For this review, take the finished solid that the model builds, in its own axes (mm). Face numbers are marked on the shaded views. A direction names the side the tool comes from. Give positions to 0.01 mm unless a question says otherwise; leave off trailing zeros. Loops run counter-clockwise (first coordinate to the right, second up) from the corner with the lowest first, then second, coordinate; pieces in that order, holes last. Notation, with made-up numbers: (-17.75, -30) - (-11.75, -30) arc R20 cw to (-11.75, -5) - close; hole circle Ø9 at (40.5, 88). An arc over 180 degrees is marked (long way). Answer in a Markdown table with one row per item.
```python
from build123d import *

# Parameters (mm, degrees)
F0_W      = 10
F0_H      = 3.5
F1_DEPTH  = 20
F2_R      = 3
F3_DEPTH  = 3.501
F6_R      = 5
F9_DEPTH  = 19
F10_DEPTH = 5
F11_R     = 5


with BuildPart() as f1:
    # F0 (on Front) → F1 (new body)
    with BuildSketch(Plane.XZ):
        with Locations((-70, 1.75)):
            Rectangle(F0_W, F0_H)
        Polygon((-65, 0), (0, 0), (0, 3.5), (0, 32), (-65, 32), (-65, 3.5), align=None)
        with Locations((5, 1.75)):
            Rectangle(F0_W, F0_H)
    extrude(amount=F1_DEPTH)

    # F2 (on face) → F3 (cut, through all)
    with BuildSketch(Plane.XY.offset(3.5)):
        with Locations((5, -10)):
            Circle(F2_R)
    f3 = extrude(amount=-F3_DEPTH, mode=Mode.SUBTRACT)

    # F5: F3 across plane
    add(f3.mirror(Plane.YZ.offset(-32.5)), mode=Mode.SUBTRACT)

    # F6
    f6_edges = [f1.edges().sort_by_distance(p)[0] for p in [
        (0, -10, 32),
        (-65, -10, 32),
    ]]
    fillet(f6_edges, radius=F6_R)

    # F8 (on face) → F9 (cut)
    with BuildSketch(Plane.XZ.offset(20)):
        with BuildLine():
            Line((-58.5, 2.5), (-6.5, 2.5))
            ThreePointArc((-6.5, 2.5), (-5.0857864376, 3.0857864376), (-4.5, 4.5))
            Line((-4.5, 4.5), (-4.5, 27.5))
            ThreePointArc((-4.5, 27.5), (-5.0857864376, 28.9142135624), (-6.5, 29.5))
            Line((-6.5, 29.5), (-58.5, 29.5))
            ThreePointArc((-58.5, 29.5), (-59.9142135624, 28.9142135624), (-60.5, 27.5))
            Line((-60.5, 27.5), (-60.5, 4.5))
            ThreePointArc((-60.5, 4.5), (-59.9142135624, 3.0857864376), (-58.5, 2.5))
        make_face()
    extrude(amount=-F9_DEPTH, mode=Mode.SUBTRACT)

    # F7 (on face) → F10 (cut)
    with BuildSketch(Plane(origin=(0, 0, 0), x_dir=(-1, 0, 0), z_dir=(0, 1, 0))):
        with BuildLine():
            Line((7.5, 4), (57.5, 4))
            ThreePointArc((57.5, 4), (58.9142135624, 4.5857864376), (59.5, 6))
            Line((59.5, 6), (59.5, 26))
            ThreePointArc((59.5, 26), (58.9142135624, 27.4142135624), (57.5, 28))
            Line((57.5, 28), (7.5, 28))
            ThreePointArc((7.5, 28), (6.0857864376, 27.4142135624), (5.5, 26))
            Line((5.5, 26), (5.5, 6))
            ThreePointArc((5.5, 6), (6.0857864376, 4.5857864376), (7.5, 4))
        make_face()
    extrude(amount=-F10_DEPTH, mode=Mode.SUBTRACT)

    # F11
    f11_edges = [f1.edges().sort_by_distance(p)[0] for p in [
        (-75, -20, 1.75),
        (-75, 0, 1.75),
        (10, -20, 1.75),
        (10, 0, 1.75),
    ]]
    fillet(f11_edges, radius=F11_R)


solid = f1.part
```
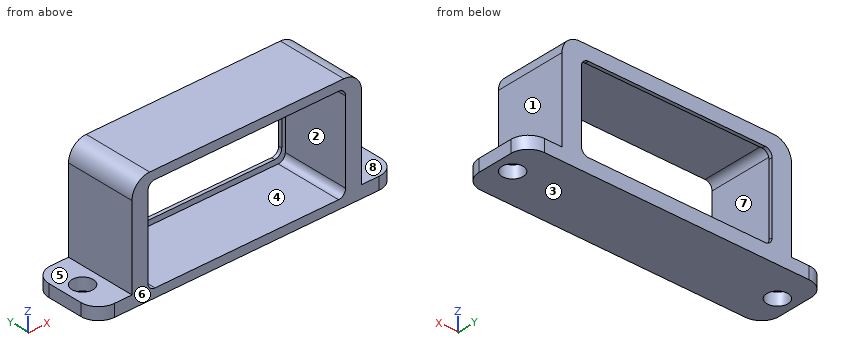
1. Mouldability with a two-part tool opening along Z and no side actions: class the marked faces 1, 2, 3 and 4 as released by +Z, released by -Z, zero draft, split by the parting line, or undercut.
Values:
| item | result |
|---|---|
| face 1 | zero draft |
| face 2 | undercut |
| face 3 | released by -Z |
| face 4 | undercut |
2. We need section A-A, the plane y = -9.25. Give the boundary of the cut face in (x, z).
Values:
| item | result |
|---|---|
| outline | (-75, 0) - (-72.9, 0) - (-72.9, 3.5) - (-75, 3.5) - close; (-67.1, 0) - (2.1, 0) - (2.1, 3.5) - (0, 3.5) - (0, 27) arc R5 ccw to (-5, 32) - (-60, 32) arc R5 ccw to (-65, 27) - (-65, 3.5) - (-67.1, 3.5) - close; (7.9, 0) - (10, 0) - (10, 3.5) - (7.9, 3.5) - close; hole (-60.5, 4.5) arc R2 ccw to (-58.5, 2.5) - (-6.5, 2.5) arc R2 ccw to (-4.5, 4.5) - (-4.5, 27.5) arc R2 ccw to (-6.5, 29.5) - (-58.5, 29.5) arc R2 ccw to (-60.5, 27.5) - close |
3. We need section C-C, the plane y = -17.5. Give the boundary of the cut face in (x, z).
Values:
| item | result |
|---|---|
| outline | (-74.33, 0) - (9.33, 0) - (9.33, 3.5) - (0, 3.5) - (0, 27) arc R5 ccw to (-5, 32) - (-60, 32) arc R5 ccw to (-65, 27) - (-65, 3.5) - (-74.33, 3.5) - close; hole (-60.5, 4.5) arc R2 ccw to (-58.5, 2.5) - (-6.5, 2.5) arc R2 ccw to (-4.5, 4.5) - (-4.5, 27.5) arc R2 ccw to (-6.5, 29.5) - (-58.5, 29.5) arc R2 ccw to (-60.5, 27.5) - close |
4. Wall thickness on line 1 (X direction, y = -18, z = 27); line 2 (Z direction, x = -47.5, y = -13.5); line 3 (Y direction, x = -70, z = 2.55): over which ranges is each line inside the solid? List them lowest first. Write a range as [from, to].
Values:
| item | result |
|---|---|
| line 1 | x = [-65, -60.5], [-4.5, 0] |
| line 2 | z = [0, 2.5], [29.5, 32] |
| line 3 | y = [-20, -13], [-7, 0] |
5. Clearance check with flat-ended pins moving along their axes: pin 1 (1 mm diameter, centred on y = -13, z = 24.5, fed in from +X); pin 2 (3 mm diameter, centred on y = -14, z = 14, fed in from -X); pin 3 (3 mm diameter, centred on x = -68, y = -9.5, fed in from +Z); pin 4 (8 mm diameter, centred on x = -55, z = 17.5, fed in from +Y). State where each tip first meets the part, or that it passes through.
Values:
| item | result |
|---|---|
| pin 1 | stops at x = 0 |
| pin 2 | stops at x = -65 |
| pin 3 | stops at z = 3.5 |
| pin 4 | passes through |
6. For the marked faces 5, 6, 7 and 8, list the 3-axis set-ups (+Z, -Z, +X, -X, +Y, -Y) from which the entire face can be reached by the end or side of a thin tool; tool diameter is ignored.
Values:
| item | result |
|---|---|
| face 5 | +Z, -X, +Y, -Y |
| face 6 | +Z, -Z, +X, -X, -Y |
| face 7 | -Y |
| face 8 | +Z, +X, +Y, -Y |
7. We need section B-B, the plane x = -49. Give the boundary of the cut face in (y, z).
Values:
| item | result |
|---|---|
| outline | (-20, 0) - (0, 0) - (0, 4) - (-1, 4) - (-1, 2.5) - (-20, 2.5) - close; (-20, 29.5) - (-1, 29.5) - (-1, 28) - (0, 28) - (0, 32) - (-20, 32) - close |
8. We need section D-D, the plane x = -1.5. Give the boundary of the cut face in (y, z).
Values:
| item | result |
|---|---|
| outline | (-20, 0) - (0, 0) - (0, 30.57) - (-20, 30.57) - close |
